For this review, take the finished solid that the model builds, in its own axes (mm). A direction names the side the tool comes from. Give positions to 0.01 mm unless a question says otherwise; leave off trailing zeros. Loops run counter-clockwise (first coordinate to the right, second up) from the corner with the lowest first, then second, coordinate; pieces in that order, holes last. Notation, with made-up numbers: (-18, 53) -> (17, 53) arc R21 cw to (17, 70) -> close; hole circle Ø1 at (-6.75, 16). An arc over 180 degrees is marked (long way). Write each question's results on one line, items separated by ' | '. Start each with the question number.
```python
from build123d import *

# Parameters (mm, degrees)
SKETCH_1_W      = 150
SKETCH_1_H      = 150
EXTRUDE_1_DEPTH = 120
SHELL_1_T       = -3


with BuildPart() as part:
    # 草图1 → 凸台-拉伸1 (new body)
    with BuildSketch(Plane.XY):
        with Locations((75, -75)):
            Rectangle(SKETCH_1_W, SKETCH_1_H)
    extrude(amount=EXTRUDE_1_DEPTH)

    # 抽壳1
    shell_1_openings = [part.faces().sort_by_distance(p)[0] for p in [
        (75, -75, 120),
    ]]
    offset(amount=SHELL_1_T, openings=shell_1_openings, kind=Kind.INTERSECTION)


solid = part.part
```
1. Draft analysis for pull direction Y (two halves, no side actions). For faces 3 (the flat face through (74, -150, 59)), 4 (the flat face through (74, -147, 61)), 5 (the flat face through (2, -41, 120)), state which applies: released by +Y, released by -Y, zero draft, split by the parting line, or undercut.
2. Machinability: for faces 1 (the flat face through (74, -3, 61)), 2 (the flat face through (150, -76, 59)), which of the approach directions +Z, -Z, +X, -X, +Y, -Y give a long, thin tool a straight path to every point of the face, cutting with its end or side? Answer none if there is none.
3. We need section B-B (y = -127). Write out the cut boundary in (x, z), plus the area to 3 significant figures.
4. For pin 1 Ø1.5 at (x, y) = (79, -94.5) entering from +Z, flat-tipped, find the tip position at first contact; note if it passes through.
5. Wall thickness on L1, parallel to X at y = -110, z = 100.5; L2, parallel to Y at x = 49, z = 72.5; L3, parallel to Z at x = 93.5, y = -120: over which ranges is each line inside the solid? List them lowest first.
6. We need section A-A (z = 91). Write out the cut boundary in (x, y).
7. We need section C-C (x = 112). Write out the cut boundary in (y, z), plus the area to 3 significant figures.
Response:
1) face 3: released by -Y | face 4: undercut | face 5: zero draft
2) face 1: +Z | face 2: +Z, -Z, +X, +Y, -Y
3) outline: (0, 0) -> (150, 0) -> (150, 120) -> (147, 120) -> (147, 3) -> (3, 3) -> (3, 120) -> (0, 120) -> close | area: 1,150 mm2
4) pin 1: stops at z = 3
5) L1: x = 0 to 3, 147 to 150 | L2: y = -150 to -147, -3 to 0 | L3: z = 0 to 3
6) outline: (0, -150) -> (150, -150) -> (150, 0) -> (0, 0) -> close; hole (3, -147) -> (147, -147) -> (147, -3) -> (3, -3) -> close
7) outline: (-150, 0) -> (0, 0) -> (0, 120) -> (-3, 120) -> (-3, 3) -> (-147, 3) -> (-147, 120) -> (-150, 120) -> close | area: 1,150 mm2
